For this review, take the finished solid that the model builds, in its own axes (mm). A direction names the side the tool comes from. Coordinates: 2 decimals unless noted, no trailing zeros. Loops run counter-clockwise (first coordinate to the right, second up) from the corner with the lowest first, then second, coordinate; pieces in that order, holes last.
1. To check wall thickness, follow probe 1 along X at (y, z) = (6.25, 4); probe 2 along Y at (x, z) = (1, -5); probe 3 along X at (y, z) = (-1.5, 5.5). State the ranges of each line that lie inside material, in increasing order.
2. Mouldability with a two-part tool opening along Y and no side actions: class faces 1 (the face through (1.726, -1.102, -9.744)), 2 (the face through (1.479, 6.528, -4.006)), 3 (the face through (3, 0, -1)), 4 (the face through (1.726, -1.887, 0.1)) as pulls with the +Y half, pulls with the -Y half, needs draft (parallel to the pull), parting line crosses it, or undercut.
3. Clearance check with flat-ended pins moving along their axes: P1, Ø2, axis at y = 4.5, z = -1, coming from the -X side; P2, Ø1, axis at x = -1.5, z = 6.5, coming from the -Y side; P3, Ø6, axis at x = -2.5, y = 6.5, coming from the +Z side; P4, Ø5, axis at x = 2, z = -6.5, coming from the +Y side. State where each tip first meets the part, or that it passes through.
4. Machinability: for faces 5 (the face through (1.726, 7.39, 5.104)), 6 (the face through (-0.944, 6.976, 3.328)), 7 (the face through (4, 2.8, 2.2)), which of the approach directions +Z, -Z, +X, -X, +Y, -Y give a long, thin tool a straight path to every point of the face, cutting with its end or side? Answer none if there is none.
5. Take a section at A-A, the plane x = 1.75. State the section outline as (y, z) points, then the cut area to 3 significant figures.
6. Take a section at B-B, the plane x = -3.5. State the section outline as (y, z) points, then the cut area to 3 significant figures.
```python
from build123d import *

# Parameters (mm, degrees)
BOSS_EXTRUDE1_DEPTH = 4
FILLET1_R           = 0.5
SHELL2_T            = -1
SKETCH2_R           = 4.25
SKETCH2_R_2         = 2.25
BOSS_EXTRUDE2_DEPTH = 8
SKETCH3_R           = 2.5
BOSS_EXTRUDE3_DEPTH = 2
FILLET2_R           = 2


with BuildPart() as part:
    # Sketch1 → Boss-Extrude1 (new body)
    with BuildSketch(Plane(origin=(0, 0, 0), x_dir=(0, 0, -1), z_dir=(1, 0, 0))):
        with BuildLine():
            ThreePointArc((2.454932738, 13.462932908), (0.124483772, 15.487279891), (-2.395757596, 13.704765785))
            ThreePointArc((-2.395757596, 13.704765785), (-5.152279099, 7.304796743), (-9.316554121, 1.717594576))
            ThreePointArc((-9.316554121, 1.717594576), (-9.70794679, -1.172591563), (-7.094283556, -2.46685917))
            ThreePointArc((-7.094283556, -2.46685917), (0, -1.887364685), (7.094283556, -2.46685917))
            ThreePointArc((7.094283556, -2.46685917), (9.763595355, -1.061195586), (9.136708277, 1.88975819))
            ThreePointArc((9.136708277, 1.88975819), (4.822059624, 7.114144441), (2.454932738, 13.462932908))
        make_face()
    extrude(amount=BOSS_EXTRUDE1_DEPTH)

    # Fillet1
    fillet1_edges = [part.edges().sort_by_distance(p)[0] for p in [
        (4, -1.887364685, 0),
        (4, -1.061195586, -9.763595355),
        (4, 7.114144441, -4.822059624),
        (4, 15.487279891, -0.124483772),
        (4, 7.304796743, 5.152279099),
        (4, -1.172591563, 9.70794679),
    ]]
    fillet(fillet1_edges, radius=FILLET1_R)

    # Shell2
    shell2_openings = [part.faces().sort_by_distance(p)[0] for p in [
        (0, 4.2016107, 0.088845764),
    ]]
    offset(amount=SHELL2_T, openings=shell2_openings, kind=Kind.INTERSECTION)

    # Sketch2 → Boss-Extrude2 (add)
    with BuildSketch(Plane.ZY.offset(-3)):
        with Locations(Location((-0.044973033, 4.389682089, 0), (0, 0, 180))):
            Circle(SKETCH2_R)
        with Locations((-0.044973033, 4.389682089)):
            Circle(SKETCH2_R_2, mode=Mode.SUBTRACT)
    extrude(amount=BOSS_EXTRUDE2_DEPTH)

    # Sketch3 → Boss-Extrude3 (add)
    with BuildSketch(Plane(origin=(4, 0, 0), x_dir=(0, 0, -1), z_dir=(1, 0, 0))):
        with Locations((0.044973661, 4.389769746)):
            Circle(SKETCH3_R)
    extrude(amount=BOSS_EXTRUDE3_DEPTH)

    # Fillet2
    fillet2_edges = [part.edges().sort_by_distance(p)[0] for p in [
        (6, 4.389769746, 2.455026339),
    ]]
    fillet(fillet2_edges, radius=FILLET2_R - 0.0001)  # a hair under: the kernel refuses the full size


solid = part.part
```
Results list:
1. probe 1: x = 3 to 4
1. probe 2: y = -2.17 to -1.17, 4.98 to 6.81
1. probe 3: x = 0 to 4
2. face 1: parting line crosses it
2. face 2: undercut
2. face 3: undercut
2. face 4: pulls with the -Y half
3. P1: stops at x = 3
3. P2: passes through
3. P3: stops at z = 6.74
3. P4: stops at y = 8.69
4. face 5: +Z, +X, -X, +Y
4. face 6: -X
4. face 7: +X
5. outline: (-2.47, -7.09) arc R2.5 ccw to (1.89, -9.14) arc R20.42 cw to (13.46, -2.45) arc R2.5 ccw to (13.7, 2.4) arc R29.87 cw to (1.72, 9.32) arc R2.5 ccw to (-2.47, 7.09) arc R43.71 cw to start; circle Ø8.5 at (4.39, -0.04); hole (-1.48, -7.26) arc R1.5 ccw to (1.13, -8.48) arc R21.42 cw to (13.27, -1.47) arc R1.5 ccw to (13.42, 1.44) arc R30.87 cw to (1.03, 8.59) arc R1.5 ccw to (-1.48, 7.26) arc R44.71 cw to start; hole circle Ø4.5 at (4.39, -0.04)
5. area: 98.9 mm2
6. outline: circle Ø8.5 at (4.39, -0.04); hole circle Ø4.5 at (4.39, -0.04)
6. area: 40.8 mm2
